```python
from build123d import *

# Parameters (mm, degrees)
F0_R     = 4.5
F2_R     = 6
F4_DEPTH = 2
F5_R     = 3.6
F6_DEPTH = 5
F7_D     = 5.2


with BuildPart() as f3:
    # F0 (on Top) → F3 section 0
    with BuildSketch(Plane.XY):
        Circle(F0_R)
    # F2 (on offset) → F3 section 1
    with BuildSketch(Plane.XY.offset(10)):
        Circle(F2_R)
    loft()

    # F4 (add): a face of the model
    f4_faces = [f3.faces().sort_by_distance(p)[0] for p in [
        (0, 0, 10),
    ]]
    extrude(f4_faces, amount=F4_DEPTH)

    # F5 (on face) → F6 (join)
    with BuildSketch(Plane.XY.offset(12)):
        Circle(F5_R)
    extrude(amount=F6_DEPTH)

    # F7 (through all)
    with Locations(Plane(origin=(0, 0, 0), x_dir=(1, 0, 0), z_dir=(0, 0, -1))):
        with Locations((0, 0)):
            Hole(F7_D / 2)


solid = f3.part
```
For this review, take the finished solid that the model builds, in its own axes (mm). A direction names the side the tool comes from. Give positions to 0.01 mm unless a question says otherwise; leave off trailing zeros. Loops run counter-clockwise (first coordinate to the right, second up) from the corner with the lowest first, then second, coordinate; pieces in that order, holes last. Notation, with made-up numbers: M 27,-0.5 L 53,-0.5 A10 ccw 53,11.5 Z; hole C 86,5.5 d11. An arc over 180 degrees is marked long. One line per item, written item: value. Start each with the question number.
Q1. Add section A-A (x = 0). Give the boundary of the cut face in (y, z), and give its area (3 significant figures).
Q2. Machinability: for faces 1 (the face through (2, -2, 0)), 2 (the face through (3.434, 1.081, 14.465)), which of the approach directions +Z, -Z, +X, -X, +Y, -Y give a long, thin tool a straight path to every point of the face, cutting with its end or side? Answer none if there is none.
Q3. For L1, parallel to Y at x = 0, z = 13; L2, parallel to Y at x = 0, z = 11.75; L3, parallel to X at y = -1, z = 13.5, list the stretches that pass through material, from the lowest coordinate up.
Q4. Add section C-C (z = 15.5). Give the boundary of the cut face in (x, y), and give its area (3 significant figures).
Q5. Clearance check with flat-ended pins moving along their axes: pin 1 Ø3 at (x, y) = (0, 0) entering from -Z; pin 2 Ø2 at (y, z) = (1.5, 3) entering from -X; pin 3 Ø4 at (x, z) = (-2, 4.5) entering from -Y; pin 4 Ø1 at (y, z) = (-1.5, 9) entering from +X. State where each tip first meets the part, or that it passes through.
Q6. Draft analysis for pull direction X (two halves, no side actions). For faces 3 (the face through (0.338, -2.578, 8.619)), 4 (the face through (2, 2, 17)), 5 (the face through (-1, -5, 4)), state which applies: released by +X, released by -X, zero draft, split by the parting line, or undercut.
Q7. Add section B-B (z = 5). Give the boundary of the cut face in (x, y).
Reply:
1. outline: M -6,10 L -4.5,0 L -2.6,0 L -2.6,17 L -3.6,17 L -3.6,12 L -6,12 Z; M 2.6,0 L 4.5,0 L 6,10 L 6,12 L 3.6,12 L 3.6,17 L 2.6,17 Z
1. area: 76.6 mm²
2. face 1: -Z, +X, -X, +Y, -Y
2. face 2: +Z
3. L1: -3.6 to -2.6, 2.6 to 3.6
3. L2: -6 to -2.6, 2.6 to 6
3. L3: -3.46 to -2.4, 2.4 to 3.46
4. outline: C 0,0 d7.2; hole C 0,0 d5.2
4. area: 19.5 mm²
5. pin 1: through
5. pin 2: x = -4.99
5. pin 3: y = -5.36
5. pin 4: x = 5.79
6. face 3: undercut
6. face 4: zero draft
6. face 5: split by the parting line
7. outline: C 0,0 d10.5; hole C 0,0 d5.2
